from build123d import *

# Parameters (mm, degrees)
F0_W         = 55.88
F0_H         = 25.4
F1_DEPTH     = 3.81
F2_W         = 46.228
F2_H         = 20.828
F3_DEPTH     = 1.778
F4_W         = 10.414
F4_H         = 9.1227373774
F5_DEPTH     = 25.4
F6_W         = 8.89
F6_H         = 15.24
F7_DEPTH     = 3.81
F8_T1_DEPTH  = 26.67
F10_W        = 8.89
F10_H        = 15.24
F11_DEPTH    = 3.81
F12_T1_DEPTH = 26.67
F13_W        = 8.89
F13_H        = 15.24
F14_DEPTH    = 3.81
F15_T1_DEPTH = 26.67
F16_W        = 8.89
F16_H        = 15.24
F17_DEPTH    = 3.81
F18_T1_DEPTH = 26.67


# Not quite as in the source:
# - a fillet or chamfer that OpenCascade refuses, or shapes differently, is made with other operations: its cross-section is extruded or revolved along the edge and cut away or added


with BuildPart() as f1:
    # F0 (on Front) → F1 (new body)
    with BuildSketch(Plane.XZ):
        with Locations((8.0322436088, 0.5406907029)):
            Rectangle(F0_W, F0_H)
    extrude(amount=F1_DEPTH)

    # F2 (on face) → F3 (join)
    with BuildSketch(Plane.XZ.offset(3.81)):
        with Locations((8.1592436088, 0.6676907029)):
            Rectangle(F2_W, F2_H)
    extrude(amount=F3_DEPTH)

    # F4 (on face) → F5 (cut)
    with BuildSketch(Plane.XZ):
        with Locations((8.0322436088, -11.3866779858)):
            Rectangle(F4_W, F4_H)
    extrude(amount=F5_DEPTH, mode=Mode.SUBTRACT)

    # F6 (on face) → F7 (join)
    with BuildSketch(Plane.XZ):
        with Locations((31.5272436088, 20.8606907029)):
            Rectangle(F6_W, F6_H)
    extrude(amount=F7_DEPTH)

    # F8: fillet of radius 4.572 on 2 edges, made by hand

    # F8_s2 → F8_t1 (cut)
    with BuildSketch(Plane.XZ.offset(-11.43)):
        with BuildLine():
            ThreePointArc((31.4002436088, 28.4806907029), (34.6331358124, 27.1415829065), (35.9722436088, 23.9086907029))
            Line((35.9722436088, 23.9086907029), (35.9722436088, 28.4806907029))
            Line((35.9722436088, 28.4806907029), (31.4002436088, 28.4806907029))
        make_face()
        with BuildLine():
            ThreePointArc((27.0822436088, 23.9086907029), (28.4213514052, 27.1415829065), (31.6542436088, 28.4806907029))
            Line((31.6542436088, 28.4806907029), (27.0822436088, 28.4806907029))
            Line((27.0822436088, 28.4806907029), (27.0822436088, 23.9086907029))
        make_face()
    extrude(amount=F8_T1_DEPTH, mode=Mode.SUBTRACT)

    # F10 (on face) → F11 (join)
    with BuildSketch(Plane.XZ):
        with Locations((-15.4627563912, 20.8606907029)):
            Rectangle(F10_W, F10_H)
    extrude(amount=F11_DEPTH)

    # F12: fillet of radius 4.572 on 2 edges, made by hand

    # F12_s2 → F12_t1 (cut)
    with BuildSketch(Plane.XZ.offset(-11.43)):
        with BuildLine():
            ThreePointArc((-19.9077563912, 23.9086907029), (-18.5686485948, 27.1415829065), (-15.3357563912, 28.4806907029))
            Line((-15.3357563912, 28.4806907029), (-19.9077563912, 28.4806907029))
            Line((-19.9077563912, 28.4806907029), (-19.9077563912, 23.9086907029))
        make_face()
        with BuildLine():
            ThreePointArc((-15.5897563912, 28.4806907029), (-12.3568641876, 27.1415829065), (-11.0177563912, 23.9086907029))
            Line((-11.0177563912, 23.9086907029), (-11.0177563912, 28.4806907029))
            Line((-11.0177563912, 28.4806907029), (-15.5897563912, 28.4806907029))
        make_face()
    extrude(amount=F12_T1_DEPTH, mode=Mode.SUBTRACT)

    # F13 (on face) → F14 (join)
    with BuildSketch(Plane.XZ):
        with Locations((31.5272436088, -19.7793092971)):
            Rectangle(F13_W, F13_H)
    extrude(amount=F14_DEPTH)

    # F15: fillet of radius 4.572 on 2 edges, made by hand

    # F15_s2 → F15_t1 (cut)
    with BuildSketch(Plane.XZ.offset(-11.43)):
        with BuildLine():
            ThreePointArc((35.9722436088, -22.8273092971), (34.6331358124, -26.0602015007), (31.4002436088, -27.3993092971))
            Line((31.4002436088, -27.3993092971), (35.9722436088, -27.3993092971))
            Line((35.9722436088, -27.3993092971), (35.9722436088, -22.8273092971))
        make_face()
        with BuildLine():
            ThreePointArc((31.6542436088, -27.3993092971), (28.4213514052, -26.0602015007), (27.0822436088, -22.8273092971))
            Line((27.0822436088, -22.8273092971), (27.0822436088, -27.3993092971))
            Line((27.0822436088, -27.3993092971), (31.6542436088, -27.3993092971))
        make_face()
    extrude(amount=F15_T1_DEPTH, mode=Mode.SUBTRACT)

    # F16 (on face) → F17 (join)
    with BuildSketch(Plane.XZ):
        with Locations((-15.4627563912, -19.7793092971)):
            Rectangle(F16_W, F16_H)
    extrude(amount=F17_DEPTH)

    # F18: fillet of radius 4.572 on 2 edges, made by hand

    # F18_s2 → F18_t1 (cut)
    with BuildSketch(Plane.XZ.offset(-11.43)):
        with BuildLine():
            ThreePointArc((-15.3357563912, -27.3993092971), (-18.5686485948, -26.0602015007), (-19.9077563912, -22.8273092971))
            Line((-19.9077563912, -22.8273092971), (-19.9077563912, -27.3993092971))
            Line((-19.9077563912, -27.3993092971), (-15.3357563912, -27.3993092971))
        make_face()
        with BuildLine():
            ThreePointArc((-11.0177563912, -22.8273092971), (-12.3568641876, -26.0602015007), (-15.5897563912, -27.3993092971))
            Line((-15.5897563912, -27.3993092971), (-11.0177563912, -27.3993092971))
            Line((-11.0177563912, -27.3993092971), (-11.0177563912, -22.8273092971))
        make_face()
    extrude(amount=F18_T1_DEPTH, mode=Mode.SUBTRACT)


solid = f1.part
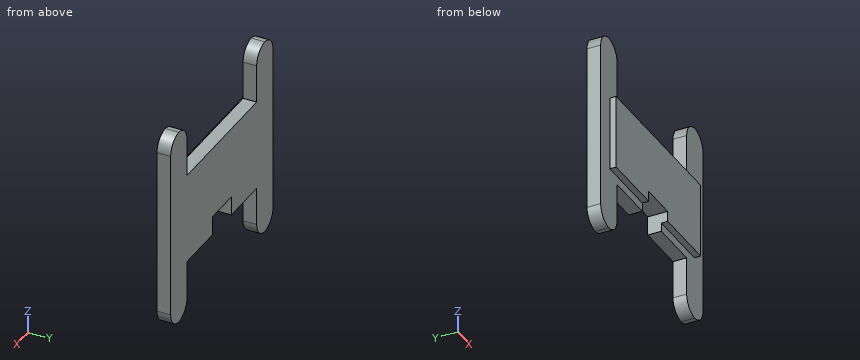
Can you work these out from the model? Positions are in its coordinate system, mm. Round coordinates to 2 decimals unless told otherwise and drop trailing zeros. Write each loop counter-clockwise with the first axis right and the second up, starting at its lowest first coordinate (ties: lowest second). Pieces come first, ordered by that corner, then holes. Notation, with made-up numbers: (61.5, -17.5) -> (92.5, -17.5) arc R22 cw to (92.5, 6.5) -> close; hole circle Ø8 at (41, 2). An arc over 180 degrees is marked (long way). Use one line per item in the form item = value. Start each with the question number.
Q1. I'm going to push flat-ended pins straight in: P1, Ø1.5, axis at x = 10.5, y = -2.5, coming from the -Z side; P2, Ø1.4, axis at y = -5, z = 5.5, coming from the +X side; P3, Ø1.9, axis at x = 10, y = -2, coming from the +Z side. Where does each tip first touch, or does it pass through?
Q2. Imagine slicing it at A-A (z = -8). Please give me the cut outline in (x, y), then the cut area to 3 significant figures.
Q3. Imagine slicing it at C-C (y = -2). Please give me the cut outline in (x, z).
Q4. Imagine slicing it at D-D (z = -14). Please give me the cut outline in (x, y), then the cut area to 3 significant figures.
Q5. Imagine slicing it at B-B (x = -10). Please give me the cut outline in (y, z), then the cut area to 3 significant figures.
Q6. If I drill on probe 1 along X at (y, z) = (-1.9, 20); probe 2 along Y at (x, z) = (26.5, -11); probe 3 along Z at (x, y) = (25.5, -4.65), over which ranges is the centre line in solid material (lowest first)? Write a range as [from, to].
Worked out:
q1.P1 = -6.83
q1.P2 = 31.27
q1.P3 = 13.24
q2.outline = (-19.91, -3.81) -> (-14.95, -3.81) -> (-14.95, -5.59) -> (2.83, -5.59) -> (2.83, 0) -> (-19.91, 0) -> close; (13.24, -5.59) -> (31.27, -5.59) -> (31.27, -3.81) -> (35.97, -3.81) -> (35.97, 0) -> (13.24, 0) -> close
q2.area = 237 mm^2
q3.outline = (-19.91, -22.83) arc R4.57 ccw to (-15.46, -27.4) arc R4.57 ccw to (-11.02, -22.83) -> (-11.02, -12.16) -> (2.83, -12.16) -> (2.83, -6.83) -> (13.24, -6.83) -> (13.24, -12.16) -> (27.08, -12.16) -> (27.08, -22.83) arc R4.57 ccw to (31.53, -27.4) arc R4.57 ccw to (35.97, -22.83) -> (35.97, 23.91) arc R4.57 ccw to (31.53, 28.48) arc R4.57 ccw to (27.08, 23.91) -> (27.08, 13.24) -> (-11.02, 13.24) -> (-11.02, 23.91) arc R4.57 ccw to (-15.46, 28.48) arc R4.57 ccw to (-19.91, 23.91) -> close
q4.outline = (-19.91, -3.81) -> (-11.02, -3.81) -> (-11.02, 0) -> (-19.91, 0) -> close; (27.08, -3.81) -> (35.97, -3.81) -> (35.97, 0) -> (27.08, 0) -> close
q4.area = 67.7 mm^2
q5.outline = (-5.59, -9.75) -> (-3.81, -9.75) -> (-3.81, -12.16) -> (0, -12.16) -> (0, 13.24) -> (-3.81, 13.24) -> (-3.81, 11.08) -> (-5.59, 11.08) -> close
q5.area = 134 mm^2
q6.probe_1 = [-19.91, -11.02], [27.08, 35.97]
q6.probe_2 = [-3.81, 0]
q6.probe_3 = [-9.75, 11.08]
